The figure shows three views and two pictorial views of one solid part (mm, origin at its lowest corner). Answer the questions. Round coordinates to 2 decimals unless told otherwise and drop trailing zeros. Order: outer loops, then holes, each group sorted by start corner. A loop starts at its lowest first (then second) coordinate and runs counter-clockwise, first axis right, second up. Notation, with made-up numbers: (78, 22) - (105, 22) arc R14 cw to (105, 39) - close; hole circle Ø9 at (4, 80). An arc over 180 degrees is marked (long way). Write item = value, one per line.
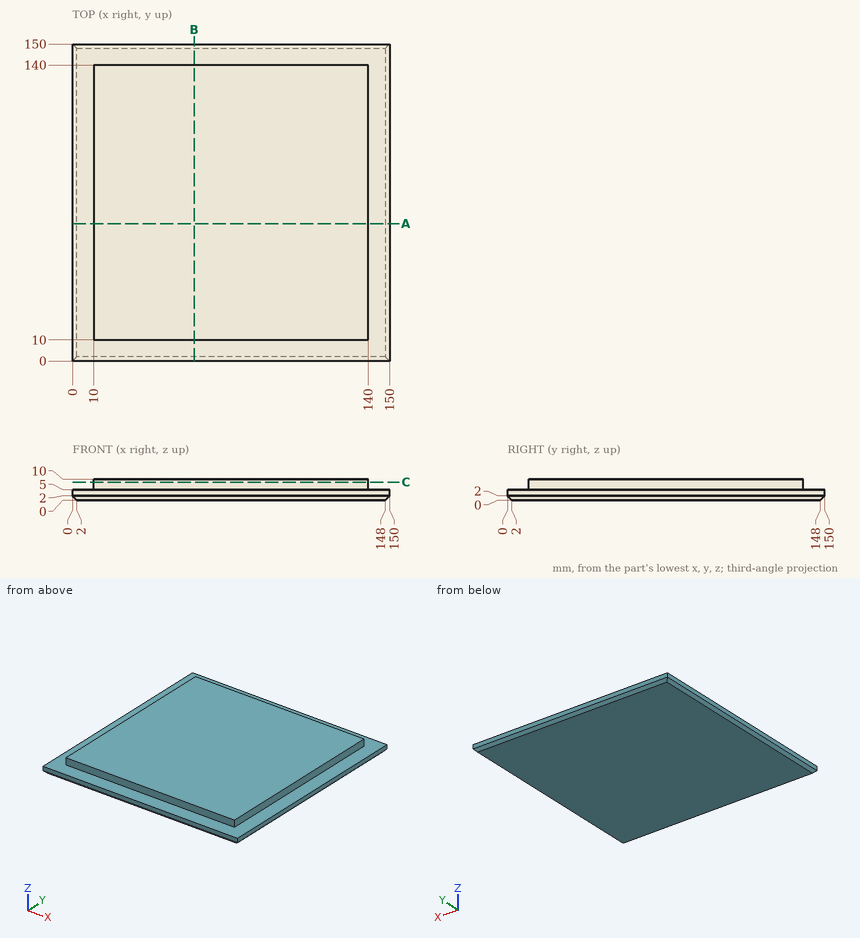
Q1. Section A-A on y = 65 is taken. Determine the outline of the cut face in (x, z).
Model answer:
outline = (0, 2) - (2, 0) - (148, 0) - (150, 2) - (150, 5) - (140, 5) - (140, 10) - (10, 10) - (10, 5) - (0, 5) - close
Q2. Section C-C on z = 8.5 is taken. Determine the outline of the cut face in (x, y), then the cut area to 3 significant figures.
Model answer:
outline = (10, 10) - (140, 10) - (140, 140) - (10, 140) - close
area = 16,900 mm^2
Q3. Find the intervals of material crossed by line 1 (X direction, y = 104, z = 7); line 2 (Z direction, x = 139, y = 7.5), in increasing order. Write a range as from..to.
Model answer:
line_1 = 10..140
line_2 = 0..5
Q4. Flat-ended cylindrical pins translate along their axes: P1, Ø4, axis at x = 89.5, z = 8.5, coming from the -Y side; P2, Ø1.5, axis at x = 75.5, z = 8, coming from the +Y side. Find the tip coordinate at first contact, or state that the pin passes through.
Model answer:
P1 = 10
P2 = 140
